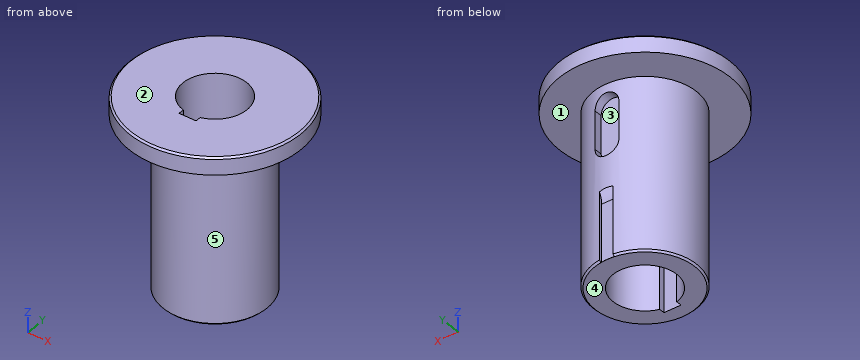
```python
from build123d import *

# Parameters (mm, degrees)
TAGLIO_ESTRUSIONE1_DEPTH = 131.385965502
TAGLIO_ESTRUSIONE5_DEPTH = 5.5
SMUSSO1_SIZE             = 1
TAGLIO_ESTRUSIONE6_DEPTH = 4


with BuildPart() as part:
    # Schizzo1 → Rivoluzione1 (revolve)
    with BuildSketch(Plane(origin=(0, 0, 0), x_dir=(0, 0, -1), z_dir=(1, 0, 0)), mode=Mode.PRIVATE) as rivoluzione1_sk:
        Polygon((-49.566192487, 49.5), (-39.566192487, 49.5), (-39.566192487, 30), (60.433807513, 30), (60.433807513, 18.5), (-49.566192487, 18.5), align=None)
    revolve(rivoluzione1_sk.sketch.rotate(Axis((0, 0, 106.615161212), (0, 0, -1)), 90), axis=Axis((0, 0, 106.615161212), (0, 0, -1)))

    # Schizzo2 → Taglio-Estrusione1 (cut, through all)
    with BuildSketch(Plane(origin=(0, 0, -60.433807513), x_dir=(-1, 0, 0), z_dir=(0, 0, -1))):
        with BuildLine():
            ThreePointArc((0, -18.5), (-2.523589416, -18.327070046), (-5, -17.811513131))
            Line((-5, -17.811513131), (-5, -21.111513131))
            Line((-5, -21.111513131), (0, -21.111513131))
            Line((0, -21.111513131), (0, -18.5))
        make_face()
        with BuildLine():
            ThreePointArc((5, -17.811513131), (2.523589416, -18.327070046), (0, -18.5))
            Line((0, -18.5), (0, -21.111513131))
            Line((0, -21.111513131), (5, -21.111513131))
            Line((5, -21.111513131), (5, -17.811513131))
        make_face()
    extrude(amount=-TAGLIO_ESTRUSIONE1_DEPTH, mode=Mode.SUBTRACT)

    # Schizzo5 → Taglio-Estrusione5 (cut)
    with BuildSketch(Plane(origin=(0, 30, 0), x_dir=(-1, 0, 0), z_dir=(0, -1, 0))):
        with BuildLine():
            Line((7, -5.566192487), (7, -27.566192487))
            ThreePointArc((7, -27.566192487), (0, -34.566192487), (-7, -27.566192487))
            Line((-7, -27.566192487), (-7, -5.566192487))
            ThreePointArc((-7, -5.566192487), (0, 1.433807513), (7, -5.566192487))
        make_face()
    extrude(amount=TAGLIO_ESTRUSIONE5_DEPTH, mode=Mode.SUBTRACT)

    # Smusso1
    smusso1_edges = [part.edges().sort_by_distance(p)[0] for p in [
        (-30, 0, -60.433807513),
        (-49.5, 0, 49.566192487),
    ]]
    chamfer(smusso1_edges, length=SMUSSO1_SIZE)

    # Schizzo7 → Taglio-Estrusione6 (cut, symmetric)
    with BuildSketch(Plane(origin=(0, 0, 0), x_dir=(0, 0, -1), z_dir=(1, 0, 0))):
        with BuildLine():
            Line((26.433807513, 51), (60.190248372, 51))
            Line((60.190248372, 51), (60.422535475, 28))
            Line((60.422535475, 28), (26.433807513, 28))
            ThreePointArc((26.433807513, 28), (14.933807513, 39.5), (26.433807513, 51))
        make_face()
    extrude(amount=TAGLIO_ESTRUSIONE6_DEPTH, both=True, mode=Mode.SUBTRACT)


solid = part.part
```
The listing builds one solid part. Answer for the finished solid, in the listing's coordinates (mm). Face numbers are marked on the shaded views. A direction names the side the tool comes from. Give positions to 0.01 mm unless a question says otherwise; leave off trailing zeros. Order: outer loops, then holes, each group sorted by start corner. A loop starts at its lowest first (then second) coordinate and runs counter-clockwise, first axis right, second up. Notation, with made-up numbers: M 60,16 L 114,16 A21 cw 114,47 Z; hole C 32.25,-40 d4. An arc over 180 degrees is marked long. Put each result on its own line as item: value. Start each with the question number.
Item 1: For a pull along X with two mould halves and no side action, classify the marked faces 3, 4 and 5 as +X half, -X half, draft (parallel to the pull), parting line (faces both ways), or undercut.
Item 2: Flat-ended cylindrical pins translate along their axes: P1, Ø5, axis at x = -13, z = 32.5, coming from the -Y side; P2, Ø3, axis at y = -5.5, z = 10, coming from the +X side; P3, Ø1.6, axis at y = -20, z = -10, coming from the +X side. Find the tip coordinate at first contact, or state that the pin passes through.
Item 3: Which of the six approach directions +Z, -Z, +X, -X, +Y, -Y give full straight-line access (tool end or side, diameter ignored) to the marked faces 1 and 2?
Item 4: Find the intervals of material crossed by line 1 along Y through (x, z) = (0, -28); line 2 along Y through (x, z) = (1, 2); line 3 along Z through (x, y) = (4.5, -31), in increasing order.
Item 5: The part is cut by section D-D, the plane z = 31. Determine the outline of the cut face in (x, y).
Item 6: The part is cut by section A-A, the plane y = 0. Determine the outline of the cut face in (x, z), and give its area (3 significant figures).
Item 7: The part is cut by section C-C, the plane z = -31. Determine the outline of the cut face in (x, y).
Answer key:
1. face 3: undercut
1. face 4: draft
1. face 5: parting line
2. P1: stops at y = -28.1
2. P2: stops at x = 29.73
2. P3: stops at x = 23.05
3. face 1: -Z
3. face 2: +Z, +X, -X, +Y, -Y
4. line 1: y = -30 to -21.11, 18.5 to 28
4. line 2: y = -29.98 to -21.11, 18.47 to 24.5
4. line 3: z = 39.57 to 49.57
5. outline: M -6.1,24.5 L -6.1,29.37 A30 ccw long 6.1,29.37 L 6.1,24.5 Z; hole M -5,-21.11 L 5,-21.11 L 5,-17.81 A18.5 ccw long -5,-17.81 Z
6. outline: M -49.5,39.57 L -30,39.57 L -30,-59.43 L -29,-60.43 L -18.5,-60.43 L -18.5,49.57 L -48.5,49.57 L -49.5,48.57 Z; M 18.5,-60.43 L 29,-60.43 L 30,-59.43 L 30,39.57 L 49.5,39.57 L 49.5,48.57 L 48.5,49.57 L 18.5,49.57 Z
6. area: 2,920 mm²
7. outline: M -4,28 L -4,29.73 A30 ccw long 4,29.73 L 4,28 Z; hole M -5,-21.11 L 5,-21.11 L 5,-17.81 A18.5 ccw long -5,-17.81 Z
